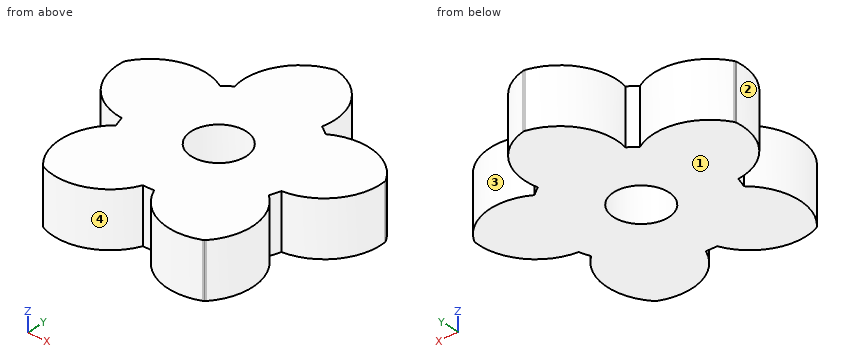
```python
from build123d import *

# Parameters (mm, degrees)
F1_DEPTH = 5
F2_R     = 2.5
F3_DEPTH = 5.001


with BuildPart() as f1:
    # F0 (on Top) → F1 (new body)
    with BuildSketch(Plane.XY):
        with BuildLine():
            ThreePointArc((7.273025, -1.831149), (7.44304, -0.922581), (7.5, 0))
            ThreePointArc((7.5, 0), (6.793658, 3.177453), (4.807679, 5.756407))
            ThreePointArc((4.807679, 5.756407), (4.408389, 6.067627), (3.989014, 6.351202))
            ThreePointArc((3.989014, 6.351202), (0, 7.5), (-3.989014, 6.351202))
            ThreePointArc((-3.989014, 6.351202), (-4.408389, 6.067627), (-4.807679, 5.756407))
            ThreePointArc((-4.807679, 5.756407), (-7.132924, 2.317627), (-7.273025, -1.831149))
            ThreePointArc((-7.273025, -1.831149), (-7.132924, -2.317627), (-6.960323, -2.793547))
            ThreePointArc((-6.960323, -2.793547), (-4.408389, -6.067627), (-0.505963, -7.482914))
            ThreePointArc((-0.505963, -7.482914), (0, -7.5), (0.505963, -7.482914))
            ThreePointArc((0.505963, -7.482914), (4.408389, -6.067627), (6.960323, -2.793547))
            ThreePointArc((6.960323, -2.793547), (7.132924, -2.317627), (7.273025, -1.831149))
        make_face()
        with BuildLine():
            ThreePointArc((4.807679, 5.756407), (6.793658, 3.177453), (7.5, 0))
            ThreePointArc((7.5, 0), (7.44304, -0.922581), (7.273025, -1.831149))
            ThreePointArc((7.273025, -1.831149), (10.763626, -0.000661), (11.919108, 3.767607))
            Line((11.919108, 3.767607), (11.888206, 3.862712))
            Line((11.888206, 3.862712), (11.857305, 3.957818))
            ThreePointArc((11.857305, 3.957818), (8.707568, 6.327235), (4.807679, 5.756407))
        make_face()
        with BuildLine():
            ThreePointArc((-3.989014, 6.351202), (0, 7.5), (3.989014, 6.351202))
            ThreePointArc((3.989014, 6.351202), (3.326772, 10.236612), (0.1, 12.5))
            Line((0.1, 12.5), (0, 12.5))
            Line((0, 12.5), (-0.1, 12.5))
            ThreePointArc((-0.1, 12.5), (-3.326772, 10.236612), (-3.989014, 6.351202))
        make_face()
        with BuildLine():
            ThreePointArc((7.428217, -10.053934), (8.708345, -6.326166), (6.960323, -2.793547))
            ThreePointArc((6.960323, -2.793547), (4.408389, -6.067627), (0.505963, -7.482914))
            ThreePointArc((0.505963, -7.482914), (3.325515, -10.237021), (7.266414, -10.171491))
            Line((7.266414, -10.171491), (7.347316, -10.112712))
            Line((7.347316, -10.112712), (7.428217, -10.053934))
        make_face()
        with BuildLine():
            ThreePointArc((-7.273025, -1.831149), (-7.132924, 2.317627), (-4.807679, 5.756407))
            ThreePointArc((-4.807679, 5.756407), (-8.707568, 6.327235), (-11.857305, 3.957818))
            Line((-11.857305, 3.957818), (-11.888206, 3.862712))
            Line((-11.888206, 3.862712), (-11.919108, 3.767607))
            ThreePointArc((-11.919108, 3.767607), (-10.763626, -0.000661), (-7.273025, -1.831149))
        make_face()
        with BuildLine():
            ThreePointArc((-7.266414, -10.171491), (-3.325515, -10.237021), (-0.505963, -7.482914))
            ThreePointArc((-0.505963, -7.482914), (-4.408389, -6.067627), (-6.960323, -2.793547))
            ThreePointArc((-6.960323, -2.793547), (-8.708345, -6.326166), (-7.428217, -10.053934))
            Line((-7.428217, -10.053934), (-7.347316, -10.112712))
            Line((-7.347316, -10.112712), (-7.266414, -10.171491))
        make_face()
    extrude(amount=F1_DEPTH)

    # F2 (on face) → F3 (cut, through all)
    with BuildSketch(Plane.XY.offset(5)):
        Circle(F2_R)
    extrude(amount=-F3_DEPTH, mode=Mode.SUBTRACT)


solid = f1.part
```
Geometry check sheet. Reference: the model listing, model coordinates, mm. Face numbers are marked on the shaded views. Round coordinates to 2 decimals unless told otherwise and drop trailing zeros. Order: outer loops, then holes, each group sorted by start corner. A loop starts at its lowest first (then second) coordinate and runs counter-clockwise, first axis right, second up. Notation, with made-up numbers: (44.25, 1) - (67.25, 1) arc R37 ccw to (67.25, 37) - close; hole circle Ø1 at (-28.5, -8.5). An arc over 180 degrees is marked (long way). Use a Markdown table: item, result. Add a question column.
1) Thickness scan on line 1 along Y through (x, z) = (0, 1.55); line 2 along Y through (x, z) = (1.75, 3.6); line 3 along X through (y, z) = (6, 2.15). Record the ranges inside material, lowest first.
2) Gauge pin test, flat ends, axial feed: P1, Ø4.5, axis at x = 0, y = 0, coming from the -Z side; P2, Ø3, axis at x = 1, z = 1, coming from the -Y side; P3, Ø3, axis at x = 3, z = 3, coming from the +Y side; P4, Ø1.5, axis at x = -8.5, z = 1.5, coming from the -Y side. Record the tip position at first contact, or that the pin passes through.
3) Section check A-A (y = 0). Record the cut outline in (x, z), then the cut area to 3 significant figures.
4) Mould release check, pull along X, two halves, no side actions. Record for the marked faces 1, 2, 3 and 4: released by +X, released by -X, zero draft, split by the parting line, or undercut.
5) Section check B-B (z = 1.1). Record the cut outline in (x, y), then the cut area to 3 significant figures.
6) Section check D-D (x = -9). Record the cut outline in (y, z).
7) Section check C-C (y = -4.25). Record the cut outline in (x, z), then the cut area to 3 significant figures.
Established:
| question | item | result |
|---|---|---|
| 1 | line 1 | -7.5 to -2.5, 2.5 to 12.5 |
| 1 | line 2 | -9.25 to -1.79, 1.79 to 11.82 |
| 1 | line 3 | -9.62 to -5.26, -4.5 to 4.5, 5.26 to 9.62 |
| 2 | P1 | through |
| 2 | P2 | y = -9.82 |
| 2 | P3 | y = 11.97 |
| 2 | P4 | y = -9.65 |
| 3 | outline | (-10.76, 0) - (-2.5, 0) - (-2.5, 5) - (-10.76, 5) - close; (2.5, 0) - (10.76, 0) - (10.76, 5) - (2.5, 5) - close |
| 3 | area | 82.6 mm2 |
| 4 | face 1 | zero draft |
| 4 | face 2 | released by -X |
| 4 | face 3 | undercut |
| 4 | face 4 | undercut |
| 5 | outline | (-11.92, 3.77) arc R5.12 ccw to (-7.27, -1.83) arc R7.5 ccw to (-6.96, -2.79) arc R5.12 ccw to (-7.43, -10.05) - (-7.35, -10.11) - (-7.27, -10.17) arc R5.12 ccw to (-0.51, -7.48) arc R7.5 ccw to (0.51, -7.48) arc R5.12 ccw to (7.27, -10.17) - (7.35, -10.11) - (7.43, -10.05) arc R5.12 ccw to (6.96, -2.79) arc R7.5 ccw to (7.27, -1.83) arc R5.12 ccw to (11.92, 3.77) - (11.89, 3.86) - (11.86, 3.96) arc R5.12 ccw to (4.81, 5.76) arc R7.5 ccw to (3.99, 6.35) arc R5.12 ccw to (0.1, 12.5) - (-0.1, 12.5) arc R5.12 ccw to (-3.99, 6.35) arc R7.5 ccw to (-4.81, 5.76) arc R5.12 ccw to (-11.86, 3.96) - (-11.89, 3.86) - close; hole circle Ø5 at (0, 0) |
| 5 | area | 328 mm2 |
| 6 | outline | (-1.37, 0) - (6.24, 0) - (6.24, 5) - (-1.37, 5) - close |
| 7 | outline | (-8.12, 0) - (8.12, 0) - (8.12, 5) - (-8.12, 5) - close |
| 7 | area | 81.2 mm2 |
